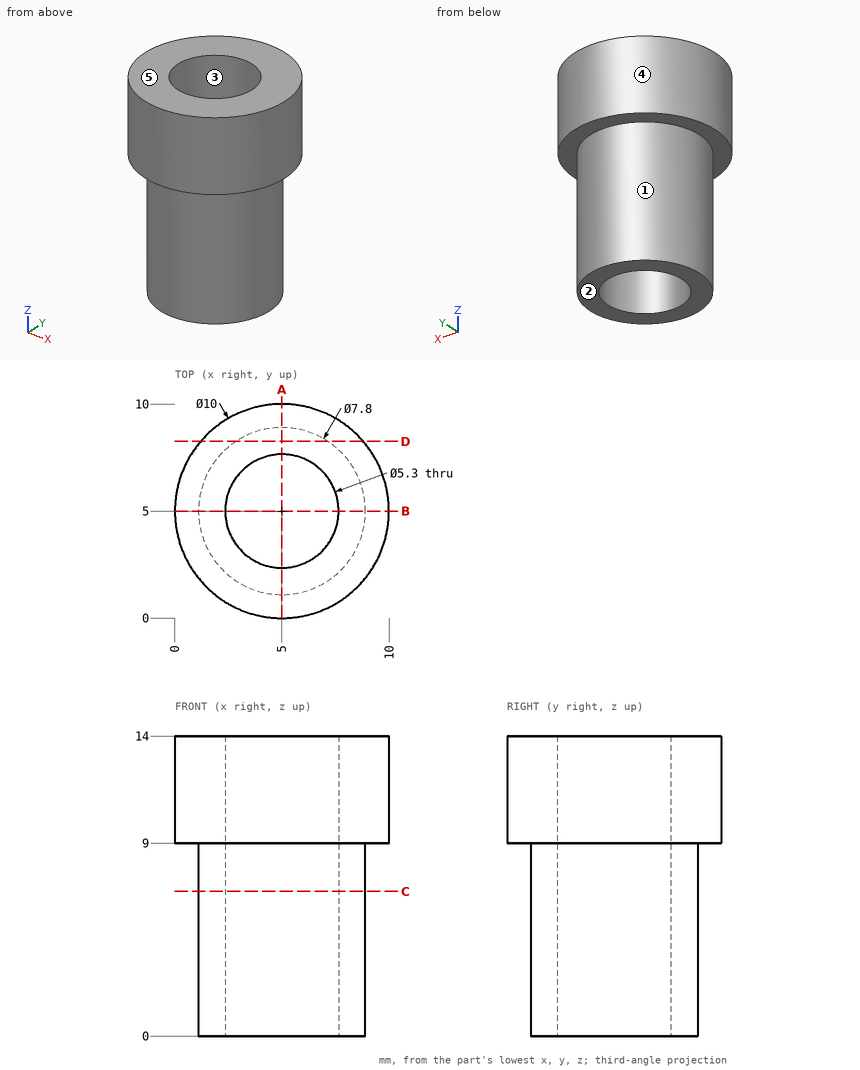
Input: dimensioned drawing with shaded views. Units: mm. Origin: part minimum x, y, z. A direction names the side the tool comes from. Coordinates: 2 decimals unless noted, no trailing zeros. Loops run counter-clockwise (first coordinate to the right, second up) from the corner with the lowest first, then second, coordinate; pieces in that order, holes last. Notation, with made-up numbers: M -25.75,55.5 L 28.25,55.5 A16 cw 28.25,80.5 Z; hole C 41.25,87 d11. An arc over 180 degrees is marked long. Put each result on its own line as item: value.
(1) Access query for the marked faces 1 and 2. Directions: +Z, -Z, +X, -X, +Y, -Y. A direction counts if a zero-diameter tool reaches every point of the face in a straight line with its end or side. Return the directions, or none.
Answer sheet:
face 1: -Z
face 2: -Z, +X, -X, +Y, -Y
(2) First-contact query: pin 1 (2 mm diameter, centred on x = 4, z = 7, fed in from +Y); pin 2 (1.5 mm diameter, centred on x = 3, z = 2.5, fed in from -Y); pin 3 (5 mm diameter, centred on x = 5, y = 5, fed in from +Z); pin 4 (6 mm diameter, centred on y = 7, z = 3, fed in from +X). Flat tips, straight axial feed; report the tip coordinate or a pass-through.
Answer sheet:
pin 1: stops at y = 8.9
pin 2: stops at y = 1.31
pin 3: passes through
pin 4: stops at x = 8.9
(3) Cut plane D-D on y = 8.25. Return the cut outline in (x, z), then the cut area to 3 significant figures.
Answer sheet:
outline: M 1.2,9 L 2.84,9 L 2.84,0 L 7.16,0 L 7.16,9 L 8.8,9 L 8.8,14 L 1.2,14 Z
area: 76.8 mm^2
(4) Cut plane A-A on x = 5. Return the cut outline in (y, z), then the cut area to 3 significant figures.
Answer sheet:
outline: M 0,9 L 1.1,9 L 1.1,0 L 2.35,0 L 2.35,14 L 0,14 Z; M 7.65,0 L 8.9,0 L 8.9,9 L 10,9 L 10,14 L 7.65,14 Z
area: 46.0 mm^2
(5) Material intervals for probe 1 along Y at (x, z) = (5, 8); probe 2 along Y at (x, z) = (5, 9.5); probe 3 along Z at (x, y) = (0.75, 6), sorted ascending.
Answer sheet:
probe 1: y = 1.1 to 2.35, 7.65 to 8.9
probe 2: y = 0 to 2.35, 7.65 to 10
probe 3: z = 9 to 14
(6) Cut plane C-C on z = 6.75. Return the cut outline in (x, y), then the cut area to 3 significant figures.
Answer sheet:
outline: C 5,5 d7.8; hole C 5,5 d5.3
area: 25.7 mm^2
(7) Draft query along Y for the marked faces 3, 4 and 5. Return one class per face: pulls with the +Y half, pulls with the -Y half, needs draft (parallel to the pull), parting line crosses it, or undercut.
Answer sheet:
face 3: undercut
face 4: parting line crosses it
face 5: needs draft
